```python
from build123d import *

# Parameters (mm, degrees)
SKETCH_1_W          = 96
SKETCH_1_H          = 56
EXTRUDE_1_DEPTH     = 35
SKETCH_5_W          = 20
SKETCH_5_H          = 54
CUT_EXTRUDE_3_DEPTH = 8
SKETCH_6_W          = 20
SKETCH_6_H          = 54
CUT_EXTRUDE_4_DEPTH = 8
SKETCH_7_W          = 12
SKETCH_7_H          = 5
CUT_EXTRUDE_5_DEPTH = 97
CUT_EXTRUDE_7_DEPTH = 3
SKETCH_9_W          = 60
SKETCH_9_H          = 15
EXTRUDE_2_DEPTH     = 12
SKETCH_10_R         = 2
CUT_EXTRUDE_8_DEPTH = 3
SKETCH_11_R         = 2.25
CUT_EXTRUDE_9_DEPTH = 15


with BuildPart() as part:
    # Эскиз1 → Бобышка-Вытянуть1 (new body)
    with BuildSketch(Plane.XY):
        with Locations((48, 28)):
            Rectangle(SKETCH_1_W, SKETCH_1_H)
    extrude(amount=EXTRUDE_1_DEPTH)

    # Эскиз5 → Вырез-Вытянуть3 (cut)
    with BuildSketch(Plane(origin=(96, 0, 0), x_dir=(0, 0, -1), z_dir=(1, 0, 0))):
        with Locations((-25, 27)):
            Rectangle(SKETCH_5_W, SKETCH_5_H)
    extrude(amount=-CUT_EXTRUDE_3_DEPTH, mode=Mode.SUBTRACT)

    # Эскиз6 → Вырез-Вытянуть4 (cut)
    with BuildSketch(Plane.ZY):
        with Locations((25, 27)):
            Rectangle(SKETCH_6_W, SKETCH_6_H)
    extrude(amount=-CUT_EXTRUDE_4_DEPTH, mode=Mode.SUBTRACT)

    # Эскиз7 → Вырез-Вытянуть5 (cut, through all)
    with BuildSketch(Plane(origin=(96, 0, 0), x_dir=(0, 0, -1), z_dir=(1, 0, 0))):
        with Locations((-6, 4)):
            Rectangle(SKETCH_7_W, SKETCH_7_H)
        with Locations((-6, 12)):
            Rectangle(SKETCH_7_W, SKETCH_7_H)
        with Locations((-6, 20)):
            Rectangle(SKETCH_7_W, SKETCH_7_H)
        with Locations((-6, 28)):
            Rectangle(SKETCH_7_W, SKETCH_7_H)
        with Locations((-6, 36)):
            Rectangle(SKETCH_7_W, SKETCH_7_H)
        with Locations((-6, 44)):
            Rectangle(SKETCH_7_W, SKETCH_7_H)
        with Locations((-6, 52)):
            Rectangle(SKETCH_7_W, SKETCH_7_H)
    extrude(amount=-CUT_EXTRUDE_5_DEPTH, mode=Mode.SUBTRACT)

    # Эскиз8 → Вырез-Вытянуть7 (cut, through all)
    with BuildSketch(Plane.XZ.offset(-54)):
        with BuildLine():
            ThreePointArc((4, 26.6), (5.6, 25), (4, 23.4))
            Line((4, 23.4), (0, 23.4))
            Line((0, 23.4), (0, 26.6))
            Line((0, 26.6), (4, 26.6))
        make_face()
        with BuildLine():
            Line((96, 26.6), (92, 26.6))
            ThreePointArc((92, 26.6), (90.4, 25), (92, 23.4))
            Line((92, 23.4), (96, 23.4))
            Line((96, 23.4), (96, 26.6))
        make_face()
    extrude(amount=-CUT_EXTRUDE_7_DEPTH, mode=Mode.SUBTRACT)

    # Эскиз9 → Бобышка-Вытянуть2 (add)
    with BuildSketch(Plane.XZ):
        with Locations((43, 25.5)):
            Rectangle(SKETCH_9_W, SKETCH_9_H)
    extrude(amount=EXTRUDE_2_DEPTH)

    # Эскиз10 → Вырез-Вытянуть8 (cut)
    with BuildSketch(Plane.XY.offset(33)):
        with Locations((18, -6)):
            Circle(SKETCH_10_R)
        with Locations((25, -6)):
            Circle(SKETCH_10_R)
        with Locations((32, -6)):
            Circle(SKETCH_10_R)
        with Locations((39, -6)):
            Circle(SKETCH_10_R)
        with Locations((46, -6)):
            Circle(SKETCH_10_R)
        with Locations((53, -6)):
            Circle(SKETCH_10_R)
        with Locations((60, -6)):
            Circle(SKETCH_10_R)
        with Locations((67, -6)):
            Circle(SKETCH_10_R)
    extrude(amount=-CUT_EXTRUDE_8_DEPTH, mode=Mode.SUBTRACT)

    # Эскиз11 → Вырез-Вытянуть9 (cut)
    with BuildSketch(Plane(origin=(0, 0, 0), x_dir=(-1, 0, 0), z_dir=(0, 0, -1))):
        with Locations((-23, 13)):
            Circle(SKETCH_11_R)
        with Locations((-73, 13)):
            Circle(SKETCH_11_R)
    extrude(amount=-CUT_EXTRUDE_9_DEPTH, mode=Mode.SUBTRACT)


solid = part.part
```
Geometry check sheet. Reference: the model listing, model coordinates, mm. A direction names the side the tool comes from. Give positions to 0.01 mm unless a question says otherwise; leave off trailing zeros. Write each loop counter-clockwise with the first axis right and the second up, starting at its lowest first coordinate (ties: lowest second). Pieces come first, ordered by that corner, then holes. Notation, with made-up numbers: (20.25, 12) -> (26.25, 12) arc R21 cw to (26.25, 16) -> close; hole circle Ø4 at (-22, 0.5). An arc over 180 degrees is marked (long way). One line per question, with ' | ' between items.
Item 1: Scan lines: line 1 along X through (y, z) = (15, 2.5); line 2 along Y through (x, z) = (60, 31); line 3 along Z through (x, y) = (60, 3). Record each from-to range of solid material in increasing order.
Determined:
line 1: 0 to 21.97, 24.03 to 71.97, 74.03 to 96 | line 2: -12 to -8, -4 to 56 | line 3: 12 to 35
Item 2: Access from +Z, -Z, +X, -X, +Y, -Y to the whole of each face (thin tool, end or side, straight path). Record for faces 1 (the flat face through (73, -6, 25)), 2 (the flat face through (25, -6, 30)), 3 (the flat face through (49, 17.5, 6)), 4 (the flat face through (23, 13, 15)).
Determined:
face 1: +Z, -Z, +X, -Y | face 2: +Z | face 3: -Z, +X, -X | face 4: -Z
Item 3: Sectioned sample at B-B, the plane z = 25. Record the boundary of the cut face in (x, y).
Determined:
outline: (5.6, 54) -> (8, 54) -> (8, 0) -> (13, 0) -> (13, -12) -> (73, -12) -> (73, 0) -> (88, 0) -> (88, 54) -> (90.4, 54) -> (90.4, 56) -> (5.6, 56) -> close
Item 4: Draft check along Y on faces 5 (the flat face through (6, 54, 25)), 6 (the flat face through (47, 8, 0)), 7 (the cylindrical face through (58, -6, 32)). Enter one of: released by +Y, released by -Y, zero draft, split by the parting line, or undercut.
Determined:
face 5: released by -Y | face 6: zero draft | face 7: undercut
Item 5: Depth check by flat-ended pin: pin 1 (5 mm diameter, centred on x = 61.5, y = 49, fed in from -Z); pin 2 (9.5 mm diameter, centred on x = 62, z = 8, fed in from -Y); pin 3 (1.5 mm diameter, centred on y = 14, z = 25, fed in from +X); pin 4 (5 mm diameter, centred on x = 53, y = -6, fed in from -Z). Enter the tip coordinate at first touch or a pass-through.
Determined:
pin 1: z = 0 | pin 2: y = 0 | pin 3: x = 88 | pin 4: z = 18
